Work out the finished part from the listing and answer in its coordinate system (mm). Face numbers are marked on the shaded views. Give positions to 0.01 mm unless a question says otherwise; leave off trailing zeros. Order: outer loops, then holes, each group sorted by start corner. A loop starts at its lowest first (then second) coordinate and runs counter-clockwise, first axis right, second up. Notation, with made-up numbers: M -22.5,33 L -0.5,33 A18 ccw -0.5,40 Z; hole C 19,-20.75 d6. An arc over 180 degrees is marked long. One line per item, written item: value.
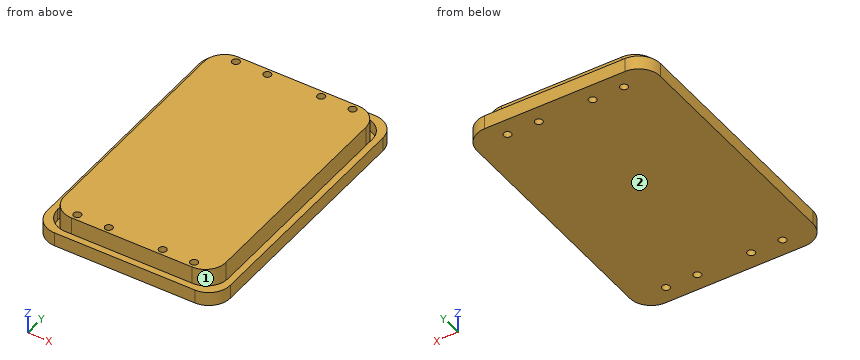
from build123d import *

# Parameters (mm, degrees)
EXTRUDE_2_DEPTH     = 6.5
EXTRUDE_3_DEPTH     = 12.7
EXTRUDE_4_DEPTH     = 1
SKETCH_5_R          = 1.78
CUT_EXTRUDE_1_DEPTH = 79.649667514


with BuildPart() as part:
    # basis → Extrude 2 (new body)
    with BuildSketch(Plane.XY):
        with BuildLine():
            ThreePointArc((32.71, 64.81), (39.781067812, 61.881067812), (42.71, 54.81))
            Line((42.71, 54.81), (42.71, -54.81))
            ThreePointArc((42.71, -54.81), (39.781067812, -61.881067812), (32.71, -64.81))
            Line((32.71, -64.81), (-32.71, -64.81))
            ThreePointArc((-32.71, -64.81), (-39.781067812, -61.881067812), (-42.71, -54.81))
            Line((-42.71, -54.81), (-42.71, 54.81))
            ThreePointArc((-42.71, 54.81), (-39.781067812, 61.881067812), (-32.71, 64.81))
            Line((-32.71, 64.81), (32.71, 64.81))
        make_face()
        with BuildLine():
            Line((-29.71, 61.81), (29.71, 61.81))
            ThreePointArc((29.71, 61.81), (36.781067812, 58.881067812), (39.71, 51.81))
            Line((39.71, 51.81), (39.71, -51.81))
            ThreePointArc((39.71, -51.81), (36.781067812, -58.881067812), (29.71, -61.81))
            Line((29.71, -61.81), (-29.71, -61.81))
            ThreePointArc((-29.71, -61.81), (-36.781067812, -58.881067812), (-39.71, -51.81))
            Line((-39.71, -51.81), (-39.71, 51.81))
            ThreePointArc((-39.71, 51.81), (-36.781067812, 58.881067812), (-29.71, 61.81))
        make_face(mode=Mode.SUBTRACT)
    extrude(amount=EXTRUDE_2_DEPTH)



with BuildPart() as body_2:
    # basis_4 → Extrude 3 (new body)
    with BuildSketch(Plane.XY):
        with BuildLine():
            Line((-28.1566, 59.81), (28.1566, 59.81))
            ThreePointArc((28.1566, 59.81), (34.911873923, 57.011873923), (37.71, 50.2566))
            Line((37.71, 50.2566), (37.71, -50.2566))
            ThreePointArc((37.71, -50.2566), (34.911873923, -57.011873923), (28.1566, -59.81))
            Line((28.1566, -59.81), (-28.1566, -59.81))
            ThreePointArc((-28.1566, -59.81), (-34.911873923, -57.011873923), (-37.71, -50.2566))
            Line((-37.71, -50.2566), (-37.71, 50.2566))
            ThreePointArc((-37.71, 50.2566), (-34.911873923, 57.011873923), (-28.1566, 59.81))
        make_face()
    extrude(amount=EXTRUDE_3_DEPTH)


with BuildPart() as part_1:
    add(part.part)

    add(body_2.part)  # Extrude 4 merges body 2
    # basis_5 → Extrude 4 (add)
    with BuildSketch(Plane.XY):
        with BuildLine():
            ThreePointArc((29.71, 61.81), (36.781067812, 58.881067812), (39.71, 51.81))
            Line((39.71, 51.81), (39.71, -51.81))
            ThreePointArc((39.71, -51.81), (36.781067812, -58.881067812), (29.71, -61.81))
            Line((29.71, -61.81), (-29.71, -61.81))
            ThreePointArc((-29.71, -61.81), (-36.781067812, -58.881067812), (-39.71, -51.81))
            Line((-39.71, -51.81), (-39.71, 51.81))
            ThreePointArc((-39.71, 51.81), (-36.781067812, 58.881067812), (-29.71, 61.81))
            Line((-29.71, 61.81), (29.71, 61.81))
        make_face()
        with BuildLine():
            ThreePointArc((-28.1566, 59.81), (-34.911873923, 57.011873923), (-37.71, 50.2566))
            Line((-37.71, 50.2566), (-37.71, -50.2566))
            ThreePointArc((-37.71, -50.2566), (-34.911873923, -57.011873923), (-28.1566, -59.81))
            Line((-28.1566, -59.81), (28.1566, -59.81))
            ThreePointArc((28.1566, -59.81), (34.911873923, -57.011873923), (37.71, -50.2566))
            Line((37.71, -50.2566), (37.71, 50.2566))
            ThreePointArc((37.71, 50.2566), (34.911873923, 57.011873923), (28.1566, 59.81))
            Line((28.1566, 59.81), (-28.1566, 59.81))
        make_face(mode=Mode.SUBTRACT)
    extrude(amount=EXTRUDE_4_DEPTH)

    # Sketch 5 → Cut-Extrude 1 (cut, through all)
    with BuildSketch(Plane(origin=(0, 0, 0), x_dir=(-1, 0, 0), z_dir=(0, 0, -1))):
        with Locations((27.21, 56.91)):
            Circle(SKETCH_5_R)
        with Locations((12.57, 56.91)):
            Circle(SKETCH_5_R)
        with Locations((-12.57, 56.91)):
            Circle(SKETCH_5_R)
        with Locations((-27.21, 56.91)):
            Circle(SKETCH_5_R)
        with Locations((27.21, -56.91)):
            Circle(SKETCH_5_R)
        with Locations((12.57, -56.91)):
            Circle(SKETCH_5_R)
        with Locations((-12.57, -56.91)):
            Circle(SKETCH_5_R)
        with Locations((-27.21, -56.91)):
            Circle(SKETCH_5_R)
    extrude(amount=-CUT_EXTRUDE_1_DEPTH, mode=Mode.SUBTRACT)


solid = part_1.part
(1) Determine the mould class of the marked faces 1 and 2 for opening direction Y: pulls with the +Y half, pulls with the -Y half, needs draft (parallel to the pull), parting line crosses it, or undercut.
Findings:
face 1: undercut
face 2: needs draft
(2) Section D-D, the plane y = 34.5 is taken. Give the vertices of the cut face in (x, z), then the cut area to 3 significant figures.
Findings:
outline: M -42.71,0 L 42.71,0 L 42.71,6.5 L 39.71,6.5 L 39.71,1 L 37.71,1 L 37.71,12.7 L -37.71,12.7 L -37.71,1 L -39.71,1 L -39.71,6.5 L -42.71,6.5 Z
area: 1,000 mm^2
(3) Given P1, Ø2, axis at y = -40.5, z = 11.5, coming from the +X side, flat-ended and moving along its own axis, determine where the tip first touches the part or whether it passes through.
Findings:
P1: stops at x = 37.71
(4) Section A-A, the plane z = 5.25 is taken. Give the number of separate pieces and of enclosed holes in the cut face, then the cut area to 3 significant figures.
Findings:
separate pieces: 2
enclosed holes: 9
area: 10,100 mm^2
(5) Section C-C, the plane y = -56.91 is taken. Give the vertices of the cut face in (x, z), then the cut area to 3 significant figures.
Findings:
outline: M -42.49,0 L -28.99,0 L -28.99,12.7 L -35.01,12.7 L -35.01,1 L -38.31,1 L -38.31,6.5 L -42.49,6.5 Z; M -25.43,0 L -14.35,0 L -14.35,12.7 L -25.43,12.7 Z; M -10.79,0 L 10.79,0 L 10.79,12.7 L -10.79,12.7 Z; M 14.35,0 L 25.43,0 L 25.43,12.7 L 14.35,12.7 Z; M 28.99,0 L 42.49,0 L 42.49,6.5 L 38.31,6.5 L 38.31,1 L 35.01,1 L 35.01,12.7 L 28.99,12.7 Z
area: 769 mm^2
(6) Section B-B, the plane x = -12.57 is taken. Give the vertices of the cut face in (y, z).
Findings:
outline: M -64.81,0 L -58.69,0 L -58.69,12.7 L -59.81,12.7 L -59.81,1 L -61.81,1 L -61.81,6.5 L -64.81,6.5 Z; M -55.13,0 L 55.13,0 L 55.13,12.7 L -55.13,12.7 Z; M 58.69,0 L 64.81,0 L 64.81,6.5 L 61.81,6.5 L 61.81,1 L 59.81,1 L 59.81,12.7 L 58.69,12.7 Z
(7) Find the intervals of material crossed by probe 1 along X at (y, z) = (18, 3); probe 2 along Y at (x, z) = (27.21, 7); probe 3 along X at (y, z) = (56, 7), in increasing order. Write a range as from..to.
Findings:
probe 1: x = -42.71..-39.71, -37.71..37.71, 39.71..42.71
probe 2: y = -59.81..-58.69, -55.13..55.13, 58.69..59.81
probe 3: x = -35.79..-28.74, -25.68..-14.1, -11.04..11.04, 14.1..25.68, 28.74..35.79
